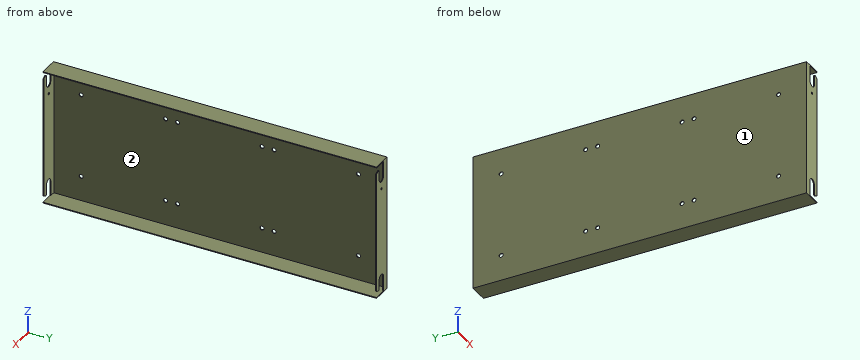
```python
from build123d import *

# Parameters (mm, degrees)
F0_W     = 415
F0_H     = 169
F1_DEPTH = 24
F2_W     = 413
F2_H     = 167
F3_DEPTH = 23
F5_DEPTH = 415.001
F6_R     = 1.5
F7_DEPTH = 415.001
F8_R     = 2.5
F9_DEPTH = 1


with BuildPart() as f1:
    # F0 (on Right) → F1 (new body)
    with BuildSketch(Plane.YZ):
        Rectangle(F0_W, F0_H)
    extrude(amount=F1_DEPTH)

    # F2 (on face) → F3 (cut)
    with BuildSketch(Plane.YZ.offset(24)):
        Rectangle(F2_W, F2_H)
    extrude(amount=-F3_DEPTH, mode=Mode.SUBTRACT)

    # F4 (on face) → F5 (cut, through all)
    with BuildSketch(Plane.XZ.offset(207.5)):
        with BuildLine():
            Line((8, -83.5), (24, -83.5))
            Line((24, -83.5), (24, -75.5))
            Line((24, -75.5), (19.5, -77.5))
            Line((19.5, -77.5), (18, -76.5))
            Line((18, -76.5), (18, -64.5))
            ThreePointArc((18, -64.5), (13, -59.5), (8, -64.5))
            Line((8, -64.5), (8, -83.5))
        make_face()
        with BuildLine():
            Line((18, 64.5), (18, 76.5))
            Line((18, 76.5), (19.5, 77.5))
            Line((19.5, 77.5), (24, 75.5))
            Line((24, 75.5), (24, 83.5))
            Line((24, 83.5), (8, 83.5))
            Line((8, 83.5), (8, 64.5))
            ThreePointArc((8, 64.5), (13, 59.5), (18, 64.5))
        make_face()
    extrude(amount=-F5_DEPTH, mode=Mode.SUBTRACT)

    # F6 (on face) → F7 (cut, through all)
    with BuildSketch(Plane.XZ.offset(207.5)):
        with Locations((12.5, 50.5)):
            Circle(F6_R)
    extrude(amount=-F7_DEPTH, mode=Mode.SUBTRACT)

    # F8 (on face) → F9 (cut, through all)
    with BuildSketch(Plane(origin=(0, 0, 0), x_dir=(0, -1, 0), z_dir=(-1, 0, 0))):
        with Locations((-172.5, 52.5)):
            Circle(F8_R)
        with Locations((-67.5, 52.5)):
            Circle(F8_R)
        with Locations((-52.5, 52.5)):
            Circle(F8_R)
        with Locations((-67.5, -52.5)):
            Circle(F8_R)
        with Locations((-172.5, -52.5)):
            Circle(F8_R)
        with Locations((-52.5, -52.5)):
            Circle(F8_R)
        with Locations((67.5, -52.5)):
            Circle(F8_R)
        with Locations((52.5, 52.5)):
            Circle(F8_R)
        with Locations((67.5, 52.5)):
            Circle(F8_R)
        with Locations((172.5, 52.5)):
            Circle(F8_R)
        with Locations((172.5, -52.5)):
            Circle(F8_R)
        with Locations((52.5, -52.5)):
            Circle(F8_R)
    extrude(amount=-F9_DEPTH, mode=Mode.SUBTRACT)


solid = f1.part
```
Can you work these out from the model? Positions are in its coordinate system, mm. Face numbers are marked on the shaded views. Round coordinates to 2 decimals unless told otherwise and drop trailing zeros. Order: outer loops, then holes, each group sorted by start corner. A loop starts at its lowest first (then second) coordinate and runs counter-clockwise, first axis right, second up.
(1) If we section it at B-B (y = 149): Please give me the cut outline in (x, z), plus the area to 3 significant figures.
Results are:
outline: (0, -84.5) - (24, -84.5) - (24, -83.5) - (1, -83.5) - (1, 83.5) - (24, 83.5) - (24, 84.5) - (0, 84.5) - close
area: 215 mm2
(2) If we section it at A-A (z = -70): Please give me the cut outline in (x, y).
Results are:
outline: (0, -207.5) - (8, -207.5) - (8, -206.5) - (1, -206.5) - (1, 206.5) - (8, 206.5) - (8, 207.5) - (0, 207.5) - close; (18, -207.5) - (24, -207.5) - (24, -206.5) - (18, -206.5) - close; (18, 206.5) - (24, 206.5) - (24, 207.5) - (18, 207.5) - close
(3) I'm going to push flat-ended pins straight in: pin 1 (2 mm diameter, centred on y = -130, z = -12, fed in from -X); pin 2 (2.5 mm diameter, centred on x = 12.5, z = 50.5, fed in from +Y); pin 3 (12 mm diameter, centred on y = 135.5, z = -48.5, fed in from +X). Where does each tip first touch, or does it pass through?
Results are:
pin 1: stops at x = 0
pin 2: passes through
pin 3: stops at x = 1
(4) If I drill on L1, parallel to Z at x = 0.55, y = 172.5; L2, parallel to Z at x = 12.5, y = 206.95; L3, parallel to Z at x = 17, y = -56.5, over which ranges is the centre line in solid material (lowest first)?
Results are:
L1: z = -84.5 to -55, -50 to 50, 55 to 84.5
L2: z = -84.5 to -83.5, -59.53 to 49, 52 to 59.53, 83.5 to 84.5
L3: z = -84.5 to -83.5, 83.5 to 84.5
(5) We'd pull the mould along Y, two halves only. Please class the marked faces 1 and 2: +Y half, -Y half, draft (parallel to the pull), parting line (faces both ways), or undercut.
Results are:
face 1: draft
face 2: undercut
(6) If we section it at C-C (z = -14): Please give me the cut outline in (x, y), plus the area to 3 significant figures.
Results are:
outline: (0, -207.5) - (24, -207.5) - (24, -206.5) - (1, -206.5) - (1, 206.5) - (24, 206.5) - (24, 207.5) - (0, 207.5) - close
area: 461 mm2
